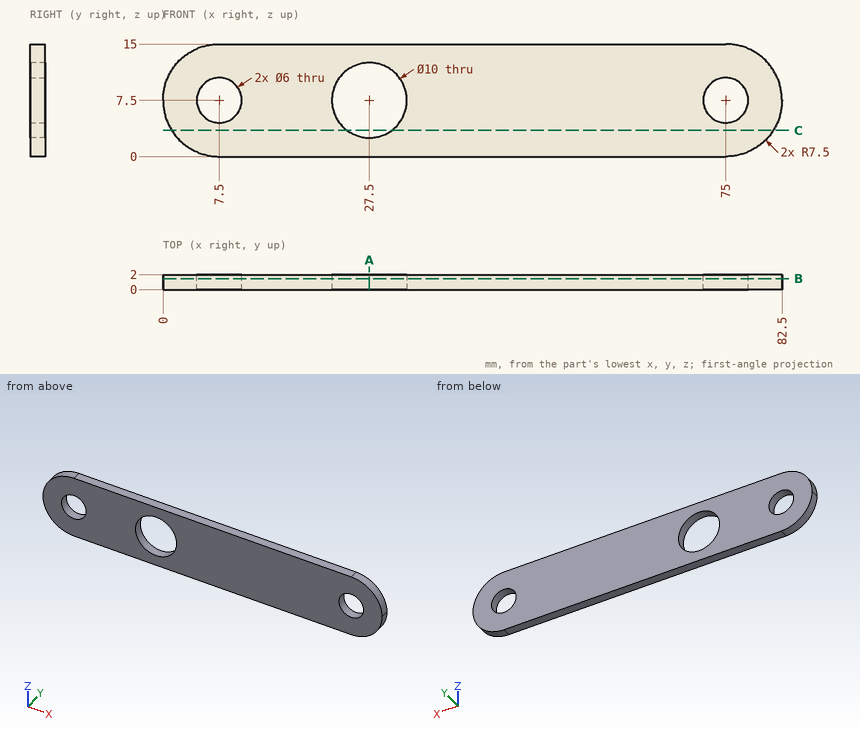
Job drawing, mm, ordinate dimensions from the low corner. One solid piece. Coordinates: 2 decimals unless noted, no trailing zeros. Order: outer loops, then holes, each group sorted by start corner. A loop starts at its lowest first (then second) coordinate and runs counter-clockwise, first axis right, second up. Notation, with made-up numbers: M 87,49 L 130,49 A19 cw 130,70 Z; hole C -35.75,36.25 d7. An arc over 180 degrees is marked long. One line per question, with ' | ' between items.
Q1. Slice it at B-B (y = 1.45). Count the separate pieces of the cut face and the enclosed holes in it, and give its area (3 significant figures).
A:
separate pieces: 1 | enclosed holes: 3 | area: 1,050 mm^2
Q2. Pin check, flat tip, straight feed: P1, Ø3.5, axis at x = 75, z = 7.5, coming from the -Y side. Stop position of the tip, or through.
A:
P1: passes through
Q3. Slice it at A-A (x = 27.5). Give the cut face in (y, z), and give its area (3 significant figures).
A:
outline: M 0,0 L 2,0 L 2,2.5 L 0,2.5 Z; M 0,12.5 L 2,12.5 L 2,15 L 0,15 Z | area: 10.0 mm^2
Q4. Slice it at C-C (z = 3.5). Give the cut face in (x, y).
A:
outline: M 1.16,0 L 24.5,0 L 24.5,2 L 1.16,2 Z; M 30.5,0 L 81.34,0 L 81.34,2 L 30.5,2 Z
Q5. Drill centre lines: line 1 (X direction, y = 0.6, z = 7.75); line 2 (Z direction, x = 75, y = 0.75); line 3 (Z direction, x = 6, y = 1.15). Where is each one in solid material? Low to high.
A:
line 1: x = 0 to 4.51, 10.49 to 22.51, 32.49 to 72.01, 77.99 to 82.5 | line 2: z = 0 to 4.5, 10.5 to 15 | line 3: z = 0.15 to 4.9, 10.1 to 14.85
